The listing builds one solid part. Answer for the finished solid, in the listing's coordinates (mm). Face numbers are marked on the shaded views. A direction names the side the tool comes from. Round coordinates to 2 decimals unless told otherwise and drop trailing zeros. Write each loop counter-clockwise with the first axis right and the second up, starting at its lowest first coordinate (ties: lowest second). Pieces come first, ordered by that corner, then holes. Notation, with made-up numbers: (37.5, 31.5) - (85.5, 31.5) arc R7 cw to (85.5, 44.5) - close; hole circle Ø4 at (25, -29). An arc over 180 degrees is marked (long way). Return JSON: item names as keys, results as strings. Group by question number.
(1) Determine the mould class of the marked faces 1, 2, 3 and 4 for opening direction X: +X half, -X half, draft (parallel to the pull), parting line (faces both ways), or undercut.
(2) Each of these flat-tipped pins is pushed along its axis until it touches: pin 1 (5 mm diameter, centred on x = -60, y = -34, fed in from +Z); pin 2 (12 mm diameter, centred on x = -1, y = -15, fed in from +Z). Where does it stop, or does it pass through?
(3) Find the intervals of material crossed by line 1 along Z through (x, y) = (32, -26), in increasing order. Write a range as [from, to].
(4) Which of the six approach directions +Z, -Z, +X, -X, +Y, -Y give full straight-line access (tool end or side, diameter ignored) to the marked faces 5 and 6?
(5) Section A-A, the plane z = 15 is taken. Give the number of separate pieces and of enclosed holes in the cut face, then the cut area to 3 significant figures.
(6) Section B-B, the plane x = 43.5 is taken. Write down the section's boundary in (y, z), then the cut area to 3 significant figures.
```python
from build123d import *

# Parameters (mm, degrees)
F1_DEPTH = 50


with BuildPart() as f1:
    # F0 (on Front) → F1 (new body)
    with BuildSketch(Plane.XZ):
        Polygon((-81.5, -22.5), (81.5, -22.5), (81.5, 22.5), (66.5, 22.5), (66.5, -7.5), (56.5, -7.5), (56.5, 22.5), (48.5, 22.5), (48.5, -7.5), (41.5, -7.5), (41.5, 22.5), (33.5, 22.5), (33.5, -7.5), (26.5, -7.5), (26.5, 22.5), (18.5, 22.5), (18.5, -7.5), (11.5, -7.5), (11.5, 22.5), (3.5, 22.5), (3.5, -7.5), (-3.5, -7.5), (-3.5, 22.5), (-11.5, 22.5), (-11.5, -7.5), (-18.5, -7.5), (-18.5, 22.5), (-26.5, 22.5), (-26.5, -7.5), (-33.5, -7.5), (-33.5, 22.5), (-41.5, 22.5), (-41.5, -7.5), (-48.5, -7.5), (-48.5, 22.5), (-56.5, 22.5), (-56.5, -7.5), (-66.5, -7.5), (-66.5, 22.5), (-81.5, 22.5), align=None)
    extrude(amount=F1_DEPTH)


solid = f1.part
```
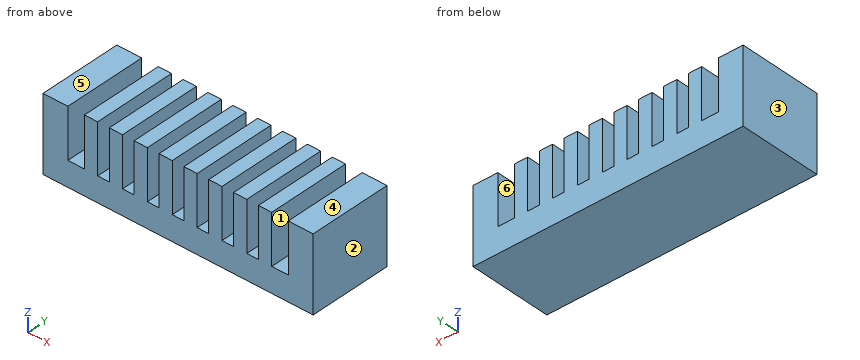
Working result:
{
 "1": {"face 1": "undercut", "face 2": "+X half", "face 3": "-X half", "face 4": "draft"},
 "2": {"pin 1": "stops at z = -7.5", "pin 2": "stops at z = 22.5"},
 "3": {"line 1": "z = [-22.5, -7.5]"},
 "4": {"face 5": "+Z, +X, -X, +Y, -Y", "face 6": "+Z, +Y, -Y"},
 "5": {"separate pieces": "10", "enclosed holes": "0", "area": "4,700 mm^2"},
 "6": {"outline": "(-50, -22.5) - (0, -22.5) - (0, -7.5) - (-50, -7.5) - close", "area": "750 mm^2"}
}
